```python
from build123d import *

# Parameters (mm, degrees)
SKETCH1_R                      = 31.115
SKETCH1_R_2                    = 28.575
EXTRUDE_THIN1_DEPTH            = 7.62
BOSS_EXTRUDE1_DEPTH            = 7.62
CUT_EXTRUDE1_REACH             = 67.161
CUT_EXTRUDE1_DIRECTION_2_DEPTH = 66.161025544
SKETCH4_W                      = 25.4
SKETCH4_H                      = 24.038818103
BOSS_EXTRUDE2_DEPTH            = 2.54
F_2_CLEARANCE_HOLE1_D          = 2.4384
F_6_32_TAPPED_HOLE1_D          = 2.7051
SKETCH9_W                      = 20.32
SKETCH9_H                      = 0.508
CUT_EXTRUDE2_DEPTH             = 66.034474296
CUT_EXTRUDE3_DEPTH             = 66.034474296
F_6_32_TAPPED_HOLE2_D          = 2.7051
F_6_32_TAPPED_HOLE2_DEPTH      = 11.176
F_6_32_TAPPED_HOLE2_TIP        = 0.81269403
F_6_32_TAPPED_HOLE3_D          = 2.7051
F_6_32_TAPPED_HOLE3_DEPTH      = 11.176
F_6_32_TAPPED_HOLE3_TIP        = 0.81269403


with BuildPart() as part:
    # Sketch1 → Extrude-Thin1 (new body)
    with BuildSketch(Plane(origin=(0, 0, 0), x_dir=(1, 0, 0), z_dir=(0, 1, 0))):
        Circle(SKETCH1_R)
        Circle(SKETCH1_R_2, mode=Mode.SUBTRACT)
    extrude(amount=EXTRUDE_THIN1_DEPTH)

    # Sketch2 → Boss-Extrude1 (add)
    with BuildSketch(Plane(origin=(0, 7.62, 0), x_dir=(1, 0, 0), z_dir=(0, 1, 0))):
        Polygon((-28.575, 0), (-28.575, -12.7), (-47.625, -12.7), (-47.625, 12.7), (-28.575, 12.7), align=None)
    extrude(amount=-BOSS_EXTRUDE1_DEPTH)

    # Sketch3 → Cut-Extrude1 (cut, up to next)
    with BuildSketch(Plane.XY.offset(12.7), mode=Mode.PRIVATE) as cut_extrude1_sk1:
        Polygon((-47.625, 0), (-43.225590949, 0), (-47.625, 7.62), align=None)
    cut_extrude1_tool1 = extrude(cut_extrude1_sk1.sketch, amount=-CUT_EXTRUDE1_REACH, mode=Mode.PRIVATE) & part.part
    add(cut_extrude1_tool1.solids().sort_by_distance((-46.15853, 2.54, 12.7))[0], mode=Mode.SUBTRACT)

    # Sketch3 → Cut-Extrude1 direction 2 (cut)
    with BuildSketch(Plane.XY.offset(12.7)):
        Polygon((-47.625, 0), (-43.225590949, 0), (-47.625, 7.62), align=None)
    extrude(amount=CUT_EXTRUDE1_DIRECTION_2_DEPTH, mode=Mode.SUBTRACT)

    # Sketch4 → Boss-Extrude2 (add)
    with BuildSketch(Plane(origin=(-32.419193212, -18.717229928, 0), x_dir=(0, 0, 1), z_dir=(-0.8660254037844413, -0.4999999999999954, 0))):
        with Locations((0, 33.632204526)):
            Rectangle(SKETCH4_W, SKETCH4_H)
    extrude(amount=-BOSS_EXTRUDE2_DEPTH)

    # #2 Clearance Hole1 (through all)
    with Locations(Plane(origin=(-30.219488686, -17.447229928, 0), x_dir=(0, 0, -1), z_dir=(0.8660254037844413, 0.4999999999999956, 0))):
        with Locations((-8.255, 41.841613577), (8.255, 41.841613577), (0, 33.586613577)):
            Hole(F_2_CLEARANCE_HOLE1_D / 2)

    # #6-32 Tapped Hole1 (through all)
    with Locations(Plane(origin=(0, 7.62, 0), x_dir=(1, 0, 0), z_dir=(0, 1, 0))):
        with Locations((-38.342060633, -8.89), (-38.342060633, 8.89)):
            Hole(F_6_32_TAPPED_HOLE1_D / 2)

    # Sketch9 → Cut-Extrude2 (cut, through all)
    with BuildSketch(Plane(origin=(0, 7.62, 0), x_dir=(1, 0, 0), z_dir=(0, 1, 0))):
        with Locations((0, 30.861)):
            Rectangle(SKETCH9_W, SKETCH9_H)
    extrude(amount=-CUT_EXTRUDE2_DEPTH, mode=Mode.SUBTRACT)

    # Sketch10 → Cut-Extrude3 (cut, through all)
    with BuildSketch(Plane(origin=(0, 7.62, 0), x_dir=(1, 0, 0), z_dir=(0, 1, 0))):
        Polygon((0, -31.115), (14.742648062, -31.115), (14.742648062, -30.607), (-16.079982159, -30.607), (-16.079982159, -31.115), align=None)
    extrude(amount=-CUT_EXTRUDE3_DEPTH, mode=Mode.SUBTRACT)

    # #6-32 Tapped Hole2
    with Locations(Plane(origin=(0, 0, -30.607), x_dir=(-1, 0, 0), z_dir=(0, 0, -1))):
        with Locations((0, 3.81)):
            Hole(F_6_32_TAPPED_HOLE2_D / 2, depth=F_6_32_TAPPED_HOLE2_DEPTH)
            with Locations((0, 0, -(F_6_32_TAPPED_HOLE2_DEPTH + F_6_32_TAPPED_HOLE2_TIP / 2))):  # 118° drill point
                Cone(0, F_6_32_TAPPED_HOLE2_D / 2, F_6_32_TAPPED_HOLE2_TIP, mode=Mode.SUBTRACT)

    # #6-32 Tapped Hole3
    with Locations(Plane.XY.offset(30.607)):
        with Locations((0, 3.81)):
            Hole(F_6_32_TAPPED_HOLE3_D / 2, depth=F_6_32_TAPPED_HOLE3_DEPTH)
            with Locations((0, 0, -(F_6_32_TAPPED_HOLE3_DEPTH + F_6_32_TAPPED_HOLE3_TIP / 2))):  # 118° drill point
                Cone(0, F_6_32_TAPPED_HOLE3_D / 2, F_6_32_TAPPED_HOLE3_TIP, mode=Mode.SUBTRACT)


solid = part.part
```
Build history of the part. All positions in model axes, mm. A direction names the side the tool comes from. Round coordinates to 2 decimals unless told otherwise and drop trailing zeros. Write each loop counter-clockwise with the first axis right and the second up, starting at its lowest first coordinate (ties: lowest second). Pieces come first, ordered by that corner, then holes. Notation, with made-up numbers: (42.25, 69) -> (100.25, 69) arc R23 cw to (100.25, 97) -> close; hole circle Ø8 at (-7.75, 39). An arc over 180 degrees is marked (long way). Put each result on its own line as item: value.
Item 1: Slice it at D-D, the plane x = -38. Give the cut face in (y, z), plus the area to 3 significant figures.
Here are the results:
outline: (0, -12.7) -> (7.62, -12.7) -> (7.62, -10.2) -> (0, -10.2) -> close; (0, -7.58) -> (7.62, -7.58) -> (7.62, 7.58) -> (0, 7.58) -> close; (0, 10.2) -> (7.62, 10.2) -> (7.62, 12.7) -> (0, 12.7) -> close
area: 154 mm^2
Item 2: Slice it at B-B, the plane y = 3.81. Give the cut face in (x, z) (3 decimals).
Here are the results:
outline: (-45.425, -12.7) -> (-28.575, -12.7) -> (-28.575, -12.313) arc R31.115 ccw to (-5.6, -30.607) -> (-1.353, -30.607) -> (-1.353, -28.543) arc R28.575 cw to (-1.353, 28.543) -> (-1.353, 30.607) -> (-5.6, 30.607) arc R31.115 ccw to (-28.575, 12.313) -> (-28.575, 12.7) -> (-45.425, 12.7) -> close; (1.353, -30.607) -> (5.6, -30.607) arc R31.115 ccw to (5.6, 30.607) -> (1.353, 30.607) -> (1.353, 28.543) arc R28.575 cw to (1.353, -28.543) -> close; hole circle Ø2.705 at (-38.342, -8.89); hole circle Ø2.705 at (-38.342, 8.89)
Item 3: Slice it at C-C, the plane z = -22. Give the cut face in (x, y).
Here are the results:
outline: (-22, 0) -> (-18.24, 0) -> (-18.24, 7.62) -> (-22, 7.62) -> close; (18.24, 0) -> (22, 0) -> (22, 7.62) -> (18.24, 7.62) -> close
Item 4: Tool access for faces 5 (the face through (-41, 6, 12.7)), 6 (the face through (-52.86, 19.19, -8.41)): list every direction of +Z, -Z, +X, -X, +Y, -Y with a clear straight run to the whole face (end or side of a thin tool).
Here are the results:
face 5: +Z, -X, +Y, -Y
face 6: none
Item 5: Slice it at A-A, the plane x = 0. Give the cut face in (y, z) (3 decimals), plus the area to 3 significant figures.
Here are the results:
outline: (0, -30.607) -> (2.457, -30.607) -> (2.457, -28.575) -> (0, -28.575) -> close; (0, 28.575) -> (2.457, 28.575) -> (2.457, 30.607) -> (0, 30.607) -> close; (5.163, -30.607) -> (7.62, -30.607) -> (7.62, -28.575) -> (5.163, -28.575) -> close; (5.163, 28.575) -> (7.62, 28.575) -> (7.62, 30.607) -> (5.163, 30.607) -> close
area: 20.0 mm^2
Item 6: Flat gauge pins, fed straight in: P1, Ø5, axis at x = -39.5, z = 2.5, coming from the -Y side; P2, Ø3, axis at x = -35.5, z = -14, coming from the +Y side. Where does each tip first touch, or does it go through?
Here are the results:
P1: stops at y = 0
P2: stops at y = 7.62
Item 7: Wall check: probe 1 along Z at (x, y) = (-50.5, 17.5); probe 2 along X at (y, z) = (3.5, 8.89); probe 3 along Z at (x, y) = (4, 4). Give the ranges that are in metal, low to high. Write a range as from..to.
Here are the results:
probe 1: z = -12.7..12.7
probe 2: x = -45.25..-39.69, -36.99..-27.16, 27.16..29.82
probe 3: z = -30.61..-28.29, 28.29..30.61
Item 8: Two-plate mould, pull along X, no slides. Class faces 1 (the face through (-54.161, 21.444, -0.178)), 2 (the face through (-39.63, 3.76, 8.48)), 3 (the face through (-29, 7.62, 2)), 4 (the face through (-47.757, 10.353, -0.968)): pulls with the +X half, pulls with the -X half, needs draft (parallel to the pull), parting line crosses it, or undercut.
Here are the results:
face 1: pulls with the -X half
face 2: undercut
face 3: needs draft
face 4: undercut
